from build123d import *

# Parameters (mm, degrees)
SKETCH1_W               = 139.7
SKETCH1_H               = 190.5
SKETCH1_W_2             = 101.6
SKETCH1_H_2             = 152.4
EXTRUDE_THIN1_DEPTH     = 152.4
CUT_EXTRUDE1_START      = -50.8
SKETCH2_W               = 101.6
SKETCH2_H               = 19.05
CUT_EXTRUDE1_DEPTH      = 50.8
SKETCH5_W               = 101.6
SKETCH5_H               = 50.8
CUT_EXTRUDE5_DEPTH      = 190.5
CUT_EXTRUDE6_DEPTH      = 228.627793777
CUT_EXTRUDE6_DEPTH_BACK = 228.627793777
SKETCH6_R               = 19.05
SKETCH7_R               = 6.35
CUT_EXTRUDE8_DEPTH      = 228.627793777
CUT_EXTRUDE2_START      = -101.6
SKETCH3_W               = 19.05
SKETCH3_H               = 127
CUT_EXTRUDE2_DEPTH      = 101.6
SKETCH4_W               = 367.241731945
SKETCH4_H               = 189.529563026
CUT_EXTRUDE4_DEPTH      = 142.24
SKETCH8_W               = 171.45
SKETCH8_H               = 101.6
BOSS_EXTRUDE1_DEPTH     = 19.05
CUT_EXTRUDE9_DEPTH      = 228.627793777
CUT_EXTRUDE9_DEPTH_BACK = 228.627793777
SKETCH9_R               = 19.05
SKETCH10_W              = 101.6
SKETCH10_H              = 25.4
BOSS_EXTRUDE2_DEPTH     = 101.6
SKETCH11_W              = 139.7
SKETCH11_H              = 50.8
CUT_EXTRUDE10_DEPTH     = 50.8


with BuildPart() as part:
    # Sketch1 → Extrude-Thin1 (new body)
    with BuildSketch(Plane(origin=(0, 0, 0), x_dir=(1, 0, 0), z_dir=(0, 1, 0))):
        Rectangle(SKETCH1_W, SKETCH1_H)
        Rectangle(SKETCH1_W_2, SKETCH1_H_2, mode=Mode.SUBTRACT)
    extrude(amount=EXTRUDE_THIN1_DEPTH)

    # Sketch2 → Cut-Extrude1 (cut)
    with BuildSketch(Plane(origin=(0, 152.4, 0), x_dir=(1, 0, 0), z_dir=(0, 1, 0)).offset(CUT_EXTRUDE1_START)):
        with Locations((0, -85.725)):
            Rectangle(SKETCH2_W, SKETCH2_H)
    extrude(amount=CUT_EXTRUDE1_DEPTH, mode=Mode.SUBTRACT)

    # Sketch5 → Cut-Extrude5 (cut)
    with BuildSketch(Plane.XY.offset(95.25)):
        with Locations((0, 127)):
            Rectangle(SKETCH5_W, SKETCH5_H)
    extrude(amount=-CUT_EXTRUDE5_DEPTH, mode=Mode.SUBTRACT)

    # Sketch6 → Cut-Extrude6 (cut, two sides: drawn at the far end of the back side and taken through both)
    with BuildSketch(Plane.ZY.offset(69.85).offset(-CUT_EXTRUDE6_DEPTH_BACK)):
        with Locations(Location((0, 38.1, 0), (0, 0, 180))):
            Circle(SKETCH6_R)
    extrude(amount=CUT_EXTRUDE6_DEPTH + CUT_EXTRUDE6_DEPTH_BACK, mode=Mode.SUBTRACT)

    # Sketch7 → Cut-Extrude8 (cut, through all)
    with BuildSketch(Plane(origin=(69.85, 0, 0), x_dir=(0, 0, -1), z_dir=(1, 0, 0))):
        with Locations((-60.452, 127)):
            Circle(SKETCH7_R)
        with Locations((60.452, 127)):
            Circle(SKETCH7_R)
    extrude(amount=-CUT_EXTRUDE8_DEPTH, mode=Mode.SUBTRACT)

    # Sketch3 → Cut-Extrude2 (cut)
    with BuildSketch(Plane.XZ.offset(CUT_EXTRUDE2_START)):
        with Locations((-60.325, 12.7)):
            Rectangle(SKETCH3_W, SKETCH3_H)
    extrude(amount=CUT_EXTRUDE2_DEPTH, mode=Mode.SUBTRACT)


with BuildPart() as body_2:
    # Mirror2: mirrored copy
    add(part.part.mirror(Plane(origin=(72.39, 0, 0), x_dir=(0, 0, 1), z_dir=(1, 0, 0))))

    # Sketch4 → Cut-Extrude4 (cut)
    with BuildSketch(Plane(origin=(72.39, 0, 0), x_dir=(0, 0, -1), z_dir=(1, 0, 0))):
        with Locations((39.035224398, 57.635218487)):
            Rectangle(SKETCH4_W, SKETCH4_H)
    extrude(amount=CUT_EXTRUDE4_DEPTH, mode=Mode.SUBTRACT)


with BuildPart() as part_1:
    add(part.part)

    # Sketch8 → Boss-Extrude1 (add)
    with BuildSketch(Plane.ZY.offset(69.85)):
        with Locations((-9.525, 50.8)):
            Rectangle(SKETCH8_W, SKETCH8_H)
    extrude(amount=-BOSS_EXTRUDE1_DEPTH)

    # Sketch9 → Cut-Extrude9 (cut, two sides: drawn at the far end of the back side and taken through both)
    with BuildSketch(Plane(origin=(69.85, 0, 0), x_dir=(0, 0, -1), z_dir=(1, 0, 0)).offset(-CUT_EXTRUDE9_DEPTH_BACK)):
        with Locations(Location((0, 38.1, 0), (0, 0, 180))):
            Circle(SKETCH9_R)
    extrude(amount=CUT_EXTRUDE9_DEPTH + CUT_EXTRUDE9_DEPTH_BACK, mode=Mode.SUBTRACT)

    # Sketch10 → Boss-Extrude2 (add)
    with BuildSketch(Plane.XZ):
        with Locations((0, -63.5)):
            Rectangle(SKETCH10_W, SKETCH10_H)
        with Locations((0, 63.5)):
            Rectangle(SKETCH10_W, SKETCH10_H)
    extrude(amount=-BOSS_EXTRUDE2_DEPTH)

    # Sketch11 → Cut-Extrude10 (cut)
    with BuildSketch(Plane(origin=(0, 152.4, 0), x_dir=(1, 0, 0), z_dir=(0, 1, 0))):
        Rectangle(SKETCH11_W, SKETCH11_H)
    extrude(amount=-CUT_EXTRUDE10_DEPTH, mode=Mode.SUBTRACT)


solid = part_1.part
Design review of the part built by this model. Coordinates are the model's own, in mm. A direction names the side the tool comes from. Give positions to 0.01 mm unless a question says otherwise; leave off trailing zeros. Loops run counter-clockwise (first coordinate to the right, second up) from the corner with the lowest first, then second, coordinate; pieces in that order, holes last. Notation, with made-up numbers: M -3,79.5 L 32,79.5 A36 ccw 32,113.5 Z; hole C 3,35.5 d6. An arc over 180 degrees is marked long. Answer as a JSON object with one key per item and string values.
Item 1: For P1, Ø22, axis at x = -11.5, z = -65, coming from the +Y side, flat-tipped, find the tip position at first contact; note if it passes through.
Output values:
{"P1": "stops at y = 101.6"}
Item 2: Mouldability with a two-part tool opening along Z and no side actions: class faces 1 (the face through (-1, 101.6, 73)), 2 (the face through (-1, 58, -95.25)), 3 (the face through (-60.458, 19.212, -2.48)) as pulls with the +Z half, pulls with the -Z half, needs draft (parallel to the pull), parting line crosses it, or undercut.
Output values:
{"face 1": "needs draft", "face 2": "pulls with the -Z half", "face 3": "undercut"}
Item 3: We need section B-B (y = 127). Count the separate pieces of the cut face and the enclosed holes in it, and give its area (3 significant figures).
Output values:
{"separate pieces": "8", "enclosed holes": "0", "area": "4,350 mm2"}
Item 4: Machinability: for faces 4 (the face through (-69.85, 75, 1)), 5 (the face through (-1, 50, 50.8)), 6 (the face through (50.8, 75, 1)), 7 (the face through (60, 101.6, 0)), which of the approach directions +Z, -Z, +X, -X, +Y, -Y give a long, thin tool a straight path to every point of the face, cutting with its end or side? Answer none if there is none.
Output values:
{"face 4": "+Z, -Z, -X, +Y, -Y", "face 5": "+Y, -Y", "face 6": "+Y", "face 7": "+X, -X, +Y"}
Item 5: We need section A-A (z = 0). State the section outline as (x, y) points, and give its area (3 significant figures).
Output values:
{"outline": "M -69.85,0 L -50.8,0 L -50.8,19.05 L -69.85,19.05 Z; M -69.85,57.15 L -50.8,57.15 L -50.8,101.6 L -69.85,101.6 Z; M 50.8,0 L 69.85,0 L 69.85,19.05 L 50.8,19.05 Z; M 50.8,57.15 L 69.85,57.15 L 69.85,101.6 L 50.8,101.6 Z", "area": "2,420 mm2"}
Item 6: We need section D-D (x = 36.5). State the section outline as (y, z) points.
Output values:
{"outline": "M 0,-95.25 L 101.6,-95.25 L 101.6,-50.8 L 0,-50.8 Z; M 0,50.8 L 101.6,50.8 L 101.6,95.25 L 0,95.25 Z"}
Item 7: Wall thickness on line 1 along Z through (x, y) = (58.5, 105); line 2 along Z through (x, y) = (30.5, 101.5); line 3 along X through (y, z) = (87, 1.5): over which ranges is each line inside the solid? List them lowest first.
Output values:
{"line 1": "z = -95.25 to -25.4, 25.4 to 95.25", "line 2": "z = -95.25 to -50.8, 50.8 to 95.25", "line 3": "x = -69.85 to -50.8, 50.8 to 69.85"}
Item 8: We need section C-C (x = 54.5). State the section outline as (y, z) points.
Output values:
{"outline": "M 0,-95.25 L 152.4,-95.25 L 152.4,-25.4 L 101.6,-25.4 L 101.6,25.4 L 152.4,25.4 L 152.4,95.25 L 0,95.25 Z; hole C 38.1,0 d38.1; hole C 127,-60.45 d12.7; hole C 127,60.45 d12.7"}
